For this review, take the finished solid that the model builds, in its own axes (mm). A direction names the side the tool comes from. Round coordinates to 2 decimals unless told otherwise and drop trailing zeros. Loops run counter-clockwise (first coordinate to the right, second up) from the corner with the lowest first, then second, coordinate; pieces in that order, holes last.
1. Consider section C-C on x = 3.05. State how many separate pieces and enclosed holes the cut face has, then the cut area to 3 significant figures.
2. Clearance check with a flat-ended pin moving along its axis: pin 1 Ø6 at (y, z) = (-101, -82) entering from -X. State where the tip first meets the part, or that it passes through.
3. Draft analysis for pull direction Y (two halves, no side actions). For faces 3 (the flat face through (4, 2, 3)), 4 (the cylindrical face through (1.97, 161.99, -207.15)), 5 (the cylindrical face through (1.97, 136.99, -177.85)), state which applies: released by +Y, released by -Y, zero draft, split by the parting line, or undercut.
4. Tool access review of faces 1 (the cylindrical face through (1.97, -58.01, -207.15)), 2 (the flat face through (0, 2, 3)): name each direction out of +Z, -Z, +X, -X, +Y, -Y from which nothing blocks a thin tool from reaching the whole face with its end or side.
5. Consider section A-A on z = 172.5. State the section outline as (x, y) points, then the cut area to 3 significant figures.
6. Consider section B-B on y = 120. State the section outline as (x, z) points, then the cut area to 3 significant figures.
7. To check wall thickness, follow line 1 along Y through (x, z) = (2.75, -95); line 2 along Y through (x, z) = (1.65, 149.75); line 3 along Z through (x, y) = (1.15, -65). State the ranges of each line that lie inside material, in increasing order.
8. Consider section D-D on z = 113. State the section outline as (x, y) points.
from build123d import *

# Parameters (mm, degrees)
EXTRUDE_1_DEPTH      = 4
SKETCH_2_R           = 1.6
SKETCH_2_W           = 90
SKETCH_2_H           = 15
CUT_EXTRUDE_1_DEPTH  = 268.097360526
SKETCH_3_R           = 2.15
CUT_EXTRUDE_3_DEPTH  = 5
SKETCH_4_R           = 2.25
CUT_EXTRUDE_5_DEPTH  = 5
SKETCH_5_W           = 35
SKETCH_5_H           = 195
CUT_EXTRUDE_6_DEPTH  = 5
SKETCH_8_R           = 1.6
CUT_EXTRUDE_8_DEPTH  = 5
SKETCH_9_R           = 1.6
CUT_EXTRUDE_9_DEPTH  = 5
SKETCH_10_R          = 1.6
SKETCH_10_W          = 41
SKETCH_10_H          = 20.5
CUT_EXTRUDE_10_DEPTH = 5
FILLET_1_R           = 10
SKETCH_11_R          = 1.6
CUT_EXTRUDE_11_DEPTH = 10


with BuildPart() as part:
    # 草图1 → 凸台-拉伸1 (new body)
    with BuildSketch(Plane(origin=(0, 0, 0), x_dir=(0, 0, -1), z_dir=(1, 0, 0))):
        with BuildLine():
            Line((200, 165), (-210, 165))
            Line((-210, 165), (-210, -165))
            Line((-210, -165), (210, -165))
            Line((210, -165), (210, 155))
            ThreePointArc((210, 155), (207.071067812, 162.071067812), (200, 165))
        make_face()
    extrude(amount=EXTRUDE_1_DEPTH)

    # 草图2 → 切除-拉伸1 (cut, through all)
    with BuildSketch(Plane(origin=(0, 0, 0), x_dir=(0, 0, -1), z_dir=(1, 0, 0))):
        with Locations((-202.5, -160)):
            Circle(SKETCH_2_R)
        with Locations((-150, -157.5)):
            Rectangle(SKETCH_2_W, SKETCH_2_H)
    cut_extrude_1 = extrude(amount=CUT_EXTRUDE_1_DEPTH, mode=Mode.SUBTRACT)

    # 镜向1: 切除-拉伸1 across plane
    add(cut_extrude_1.mirror(Plane.XY), mode=Mode.SUBTRACT)

    # 草图3 → 切除-拉伸3 (cut)
    with BuildSketch(Plane(origin=(4, 0, 0), x_dir=(0, 0, -1), z_dir=(1, 0, 0))):
        with Locations((95, 155)):
            Circle(SKETCH_3_R)
        with Locations((-95, 155)):
            Circle(SKETCH_3_R)
        with Locations(Location((95, -155, 0), (0, 0, 180))):
            Circle(SKETCH_3_R)
        with Locations(Location((-95, -155, 0), (0, 0, 180))):
            Circle(SKETCH_3_R)
        with Locations((-95, 0)):
            Circle(SKETCH_3_R)
        with Locations((95, 0)):
            Circle(SKETCH_3_R)
    extrude(amount=-CUT_EXTRUDE_3_DEPTH, mode=Mode.SUBTRACT)

    # 草图4 → 切除-拉伸5 (cut)
    with BuildSketch(Plane(origin=(4, 0, 0), x_dir=(0, 0, -1), z_dir=(1, 0, 0))):
        with Locations((203.5, 153.5)):
            Circle(SKETCH_4_R)
        with Locations((161.5, 153.5)):
            Circle(SKETCH_4_R)
    extrude(amount=-CUT_EXTRUDE_5_DEPTH, mode=Mode.SUBTRACT)

    # 草图5 → 切除-拉伸6 (cut)
    with BuildSketch(Plane(origin=(4, 0, 0), x_dir=(0, 0, -1), z_dir=(1, 0, 0))):
        with Locations((192.5, 42.5)):
            Rectangle(SKETCH_5_W, SKETCH_5_H)
    extrude(amount=-CUT_EXTRUDE_6_DEPTH, mode=Mode.SUBTRACT)

    # 草图8 → 切除-拉伸8 (cut)
    with BuildSketch(Plane.ZY):
        with Locations((-180, -65)):
            Circle(SKETCH_8_R)
        with Locations((-110.681235188, -74.742117067)):
            Circle(SKETCH_8_R)
        with Locations((-41.362470376, -84.484234134)):
            Circle(SKETCH_8_R)
        with Locations((27.956294436, -94.226351202)):
            Circle(SKETCH_8_R)
        with Locations((97.275059248, -103.968468269)):
            Circle(SKETCH_8_R)
        with Locations((166.59382406, -113.710585336)):
            Circle(SKETCH_8_R)
    extrude(amount=-CUT_EXTRUDE_8_DEPTH, mode=Mode.SUBTRACT)

    # 草图9 → 切除-拉伸9 (cut)
    with BuildSketch(Plane(origin=(4, 0, 0), x_dir=(0, 0, -1), z_dir=(1, 0, 0))):
        with Locations((-198, 160)):
            Circle(SKETCH_9_R)
        with Locations((-123, 160)):
            Circle(SKETCH_9_R)
    extrude(amount=-CUT_EXTRUDE_9_DEPTH, mode=Mode.SUBTRACT)

    # 草图10 → 切除-拉伸10 (cut)
    with BuildSketch(Plane(origin=(4, 0, 0), x_dir=(0, 0, -1), z_dir=(1, 0, 0))):
        with Locations((-199.25, -129.75)):
            Circle(SKETCH_10_R)
        with Locations((-199.25, -139.75)):
            Circle(SKETCH_10_R)
        with Locations(Location((-149.75, -139.75, 0), (0, 0, 180))):
            Circle(SKETCH_10_R)
        with Locations(Location((-149.75, -129.75, 0), (0, 0, 180))):
            Circle(SKETCH_10_R)
        with Locations((-174.5, -134.75)):
            Rectangle(SKETCH_10_W, SKETCH_10_H)
    extrude(amount=-CUT_EXTRUDE_10_DEPTH, mode=Mode.SUBTRACT)

    # 圆角1
    fillet_1_edges = [part.edges().sort_by_distance(p)[0] for p in [
        (2, -55, -210),
        (2, 140, -175),
        (2, 140, -210),
    ]]
    fillet(fillet_1_edges, radius=FILLET_1_R)

    # 草图11 → 切除-拉伸11 (cut)
    with BuildSketch(Plane(origin=(4, 0, 0), x_dir=(0, 0, -1), z_dir=(1, 0, 0))):
        with Locations((202.5, -70)):
            Circle(SKETCH_11_R)
    extrude(amount=-CUT_EXTRUDE_11_DEPTH, mode=Mode.SUBTRACT)


solid = part.part
Resolved:
1. separate pieces: 1
1. enclosed holes: 24
1. area: 128,000 mm2
2. pin 1: stops at x = 0
3. face 3: zero draft
3. face 4: released by +Y
3. face 5: undercut
4. face 1: -Z, +X, -X
4. face 2: +Z, -Z, -X, +Y, -Y
5. outline: (0, -150) - (4, -150) - (4, -145) - (0, -145) - close; (0, -124.5) - (4, -124.5) - (4, 165) - (0, 165) - close
5. area: 1,180 mm2
6. outline: (0, -175) - (4, -175) - (4, 210) - (0, 210) - close
6. area: 1,540 mm2
7. line 1: y = -165 to -157.15, -152.85 to -2.15, 2.15 to 152.85, 157.15 to 165
7. line 2: y = -150 to -141.35, -138.15 to -131.35, -128.15 to 165
7. line 3: z = -210 to -181.6, -178.4 to 210
8. outline: (0, -150) - (4, -150) - (4, 165) - (0, 165) - close
